The model under review builds one solid part; all positions refer to its coordinate system, in mm. A direction names the side the tool comes from. Give positions to 0.01 mm unless a question says otherwise; leave off trailing zeros. Order: outer loops, then holes, each group sorted by start corner. A loop starts at its lowest first (then second) coordinate and runs counter-clockwise, first axis right, second up. Notation, with made-up numbers: (47, 73) -> (59, 73) arc R15 cw to (59, 92) -> close; hole circle Ø4 at (40.25, 6.25). An arc over 180 degrees is marked (long way). Use one line per item in the form item = value.
```python
from build123d import *

# Parameters (mm, degrees)
BOSS_EXTRUDE1_DEPTH  = 6.35
FILLET1_R            = 2.54
BOSS_EXTRUDE2_DEPTH  = 6.35
FILLET2_R            = 2.54
FILLET2_OF_MIRROR1_R = 2.54


with BuildPart() as part:
    # Sketch1 → Boss-Extrude1 (new body)
    with BuildSketch(Plane.XY):
        with BuildLine():
            Line((-100.0379, 0), (-119.0879, 0))
            Line((-119.0879, 0), (-119.0879, 3.175))
            Line((-119.0879, 3.175), (-103.164054309, 3.175))
            ThreePointArc((-103.164054309, 3.175), (0, 103.2129), (103.164054309, 3.175))
            Line((103.164054309, 3.175), (119.0879, 3.175))
            Line((119.0879, 3.175), (119.0879, 0))
            Line((119.0879, 0), (100.0379, 0))
            ThreePointArc((100.0379, 0), (0, 100.0379), (-100.0379, 0))
        make_face()
    extrude(amount=BOSS_EXTRUDE1_DEPTH)

    # Fillet1
    fillet1_edges = [part.edges().sort_by_distance(p)[0] for p in [
        (-103.164054309, 3.175, 3.175),
        (103.164054309, 3.175, 3.175),
    ]]
    fillet(fillet1_edges, radius=FILLET1_R)

    # Sketch2 → Boss-Extrude2 (add)
    with BuildSketch(Plane.XY.offset(6.35)):
        with BuildLine():
            Line((-100.84827624, 87.377892058), (-79.406290546, 65.935906365))
            Line((-79.406290546, 65.935906365), (-70.737477466, 70.737477466))
            Line((-70.737477466, 70.737477466), (-65.935906365, 79.406290546))
            Line((-65.935906365, 79.406290546), (-87.377892058, 100.84827624))
            ThreePointArc((-87.377892058, 100.84827624), (-100.84827624, 100.84827624), (-100.84827624, 87.377892058))
        make_face()
        Polygon((-94.617411453, 85.637155332), (-85.637155332, 94.617411453), (-72.166771151, 81.147027272), (-81.147027272, 72.166771151), align=None, mode=Mode.SUBTRACT)
    boss_extrude2 = extrude(amount=-BOSS_EXTRUDE2_DEPTH)

    # Fillet2
    fillet2_edges = [part.edges().sort_by_distance(p)[0] for p in [
        (-65.935906365, 79.406290546, 3.175),
        (-79.406290546, 65.935906365, 3.175),
        (-94.617411453, 85.637155332, 3.175),
        (-85.637155332, 94.617411453, 3.175),
        (-72.166771151, 81.147027272, 3.175),
        (-81.147027272, 72.166771151, 3.175),
    ]]
    fillet(fillet2_edges, radius=FILLET2_R)

    # Sketch3 → 1/4 Clearance Hole1 (revolve, cut)
    with BuildSketch(Plane(origin=(-94.113084149, 94.113084149, 6.35), x_dir=(0, -1, 0), z_dir=(1, 0, 0))):
        Polygon((0, 0), (0, 27.429827343), (3.3782, 25.4), (3.3782, 0), align=None)
    f_1_4_clearance_hole1 = revolve(axis=Axis((-94.113084149, 94.113084149, 12.7), (0, 0, -1)), mode=Mode.SUBTRACT)

    # Sketch5 → #6 Clearance Hole1 (revolve, cut)
    with BuildSketch(Plane(origin=(-112.343132364, 3.175, 3.175), x_dir=(0, 0, 1), z_dir=(1, 0, 0))):
        Polygon((0, 0), (0, 26.540824014), (1.89865, 25.4), (1.89865, 0), align=None)
    f_6_clearance_hole1 = revolve(axis=Axis((-112.343132364, 9.525, 3.175), (0, -1, 0)), mode=Mode.SUBTRACT)

    # Mirror1: Boss-Extrude2, 1/4 Clearance Hole1, #6 Clearance Hole1 across plane
    add(boss_extrude2.mirror(Plane(origin=(0, 0, 0), x_dir=(0, 0, 1), z_dir=(1, 0, 0))))
    add(f_1_4_clearance_hole1.mirror(Plane(origin=(0, 0, 0), x_dir=(0, 0, 1), z_dir=(1, 0, 0))), mode=Mode.SUBTRACT)
    add(f_6_clearance_hole1.mirror(Plane(origin=(0, 0, 0), x_dir=(0, 0, 1), z_dir=(1, 0, 0))), mode=Mode.SUBTRACT)

    # Fillet2 of Mirror1
    fillet2_of_mirror1_edges = [part.edges().sort_by_distance(p)[0] for p in [
        (65.935906365, 79.406290546, 3.175),
        (79.406290546, 65.935906365, 3.175),
        (94.617411453, 85.637155332, 3.175),
        (85.637155332, 94.617411453, 3.175),
        (72.166771151, 81.147027272, 3.175),
        (81.147027272, 72.166771151, 3.175),
    ]]
    fillet(fillet2_of_mirror1_edges, radius=FILLET2_OF_MIRROR1_R)


solid = part.part
```
1. Add section C-C on y = 38.5. Give the boundary of the cut face in (x, z), then the cut area to 3 significant figures.
Values:
outline = (-95.76, 0) -> (-92.33, 0) -> (-92.33, 6.35) -> (-95.76, 6.35) -> close; (92.33, 0) -> (95.76, 0) -> (95.76, 6.35) -> (92.33, 6.35) -> close
area = 43.6 mm^2
2. Add section A-A on y = 13. Give the boundary of the cut face in (x, z).
Values:
outline = (-102.39, 0) -> (-99.19, 0) -> (-99.19, 6.35) -> (-102.39, 6.35) -> close; (99.19, 0) -> (102.39, 0) -> (102.39, 6.35) -> (99.19, 6.35) -> close
3. Tool access review of faces 4 (the face through (-96.66, 36.19, 3.13)), 5 (the face through (76.619, 76.695, 3.219)), 6 (the face through (-111, 3.175, 5)): name each direction out of +Z, -Z, +X, -X, +Y, -Y from which nothing blocks a thin tool from reaching the whole face with its end or side.
Values:
face_4 = +Z, -Z, -X
face_5 = +Z, -Z
face_6 = +Z, -Z, -X, +Y
4. Add section B-B on x = 0. Give the boundary of the cut face in (y, z), then the cut area to 3 significant figures.
Values:
outline = (100.04, 0) -> (103.21, 0) -> (103.21, 6.35) -> (100.04, 6.35) -> close
area = 20.2 mm^2
5. Add section D-D on x = -28. Give the boundary of the cut face in (y, z).
Values:
outline = (96.04, 0) -> (99.34, 0) -> (99.34, 6.35) -> (96.04, 6.35) -> close
6. For pin 1 Ø3 at (y, z) = (59, 2) entering from -X; pin 2 Ø3 at (x, z) = (115, 2) entering from +Y (3 decimals); pin 3 Ø2 at (y, z) = (32.5, 5.5) entering from +X, all flat-tipped, find the tip position at first contact; note any pin that passes through.
Values:
pin_1 = -85.71
pin_2 = 3.175
pin_3 = 98.29
7. The part is to be moulded in two halves that separate along X. For faces 1 (the face through (-76.619, 76.695, 3.219)), 2 (the face through (91.08, 77.61, 3.22)), 3 (the face through (111, 3.175, 5)), say which applies: +X half, -X half, draft (parallel to the pull), parting line (faces both ways), or undercut.
Values:
face_1 = undercut
face_2 = +X half
face_3 = draft
8. For L1, parallel to X at y = 81.5, z = 0.5; L2, parallel to X at y = 54, z = 4; L3, parallel to X at y = 30, z = 1.25, list the stretches that pass through material, from the lowest coordinate up.
Values:
L1 = -94.97 to -90.48, -73.24 to -68.03, -63.33 to -58.01, 58.01 to 63.33, 68.03 to 73.24, 90.48 to 94.97
L2 = -87.96 to -84.21, 84.21 to 87.96
L3 = -98.76 to -95.43, 95.43 to 98.76
